Design review of the part built by this model. Coordinates are the model's own, in mm. A direction names the side the tool comes from. Give positions to 0.01 mm unless a question says otherwise; leave off trailing zeros. Loops run counter-clockwise (first coordinate to the right, second up) from the corner with the lowest first, then second, coordinate; pieces in that order, holes last. Notation, with made-up numbers: (4, 37) - (21, 37) arc R20 ccw to (21, 62) - close; hole circle Ø3 at (-3.75, 7.5). An arc over 180 degrees is marked (long way). One line per item, written item: value. Start each with the question number.
```python
from build123d import *

# Parameters (mm, degrees)
SKETCH1_R           = 1.4
BOSS_EXTRUDE1_DEPTH = 3


with BuildPart() as part:
    # Sketch1 → Boss-Extrude1 (new body)
    with BuildSketch(Plane(origin=(0, 0, 0), x_dir=(1, 0, 0), z_dir=(0, 1, 0))):
        with BuildLine():
            Line((-6.037453791, -13.924683413), (-12.047861431, -7.914275773))
            ThreePointArc((-12.047861431, -7.914275773), (-12.926541087, -5.792955429), (-12.047861431, -3.671635086))
            Line((-12.047861431, -3.671635086), (8.458235223, 16.834461569))
            ThreePointArc((8.458235223, 16.834461569), (10.579555567, 17.713141225), (12.700875911, 16.834461569))
            Line((12.700875911, 16.834461569), (18.711283551, 10.824053929))
            ThreePointArc((18.711283551, 10.824053929), (19.418390332, 10.53116071), (20.125497113, 10.824053929))
            Line((20.125497113, 10.824053929), (25.075244581, 15.773801397))
            Line((25.075244581, 15.773801397), (17.606467502, 23.242578477))
            ThreePointArc((17.606467502, 23.242578477), (15.984350757, 24.326442233), (14.070933596, 24.707044571))
            Line((14.070933596, 24.707044571), (7.088177538, 24.707044571))
            ThreePointArc((7.088177538, 24.707044571), (5.174760376, 24.326442233), (3.552643632, 23.242578477))
            Line((3.552643632, 23.242578477), (-18.455978339, 1.233956505))
            ThreePointArc((-18.455978339, 1.233956505), (-19.539842096, -0.388160239), (-19.920444433, -2.301577401))
            Line((-19.920444433, -2.301577401), (-19.920444433, -9.284333458))
            ThreePointArc((-19.920444433, -9.284333458), (-19.539842096, -11.19775062), (-18.455978339, -12.819867364))
            Line((-18.455978339, -12.819867364), (-10.987201259, -20.288644444))
            Line((-10.987201259, -20.288644444), (-6.037453791, -15.338896975))
            ThreePointArc((-6.037453791, -15.338896975), (-5.744560572, -14.631790194), (-6.037453791, -13.924683413))
        make_face()
        with Locations((18.711283551, 16.480908178)):
            Circle(SKETCH1_R, mode=Mode.SUBTRACT)
        with Locations((2.447827583, 16.480908178)):
            Circle(SKETCH1_R, mode=Mode.SUBTRACT)
        with Locations((-11.69430804, 2.338772554)):
            Circle(SKETCH1_R, mode=Mode.SUBTRACT)
        with Locations((-11.69430804, -13.924683413)):
            Circle(SKETCH1_R, mode=Mode.SUBTRACT)
    extrude(amount=BOSS_EXTRUDE1_DEPTH)


solid = part.part
```
(1) Take a section at D-D on z = 8.5. State the section outline as (x, y) points.
(2) Take a section at C-C on y = 0.5. State the section outline as (x, z) points.
(3) Draft analysis for pull direction Z (two halves, no side actions). For faces 1 (the flat face through (-14.774, 1.479, 16.502)), 2 (the cylindrical face through (-12.926, 1.479, 5.826)), 3 (the cylindrical face through (-13.093, 1.479, -2.4)), 4 (the flat face through (-3, 3, -7)), state which applies: pulls with the +Z half, pulls with the -Z half, needs draft (parallel to the pull), parting line crosses it, or undercut.
(4) Take a section at A-A on x = 19.5. State the section outline as (y, z) points.
(5) Take a section at B-B on z = -3. State the section outline as (x, y) points, and give its area (3 significant figures).
(6) For pin 1 Ø4.5 at (x, z) = (-11.69, 13.92) entering from +Y; pin 2 Ø1.7 at (x, z) = (2.45, -16.48) entering from +Y, all flat-tipped, find the tip position at first contact; note any pin that passes through.
(7) To check wall thickness, follow L1, parallel to X at y = 0.2, z = -15.5; L2, parallel to X at y = 1.1, z = -1.5; L3, parallel to Z at x = 18, y = 0.6. State the ranges of each line that lie inside material, in increasing order. Write a range as from..to.
(8) Machinability: for faces 5 (the flat face through (-1.938, 1.479, -6.438)), 6 (the flat face through (15.664, 1.479, -13.871)), 7 (the flat face through (-9, 1.48, 10.96)), which of the approach directions +Z, -Z, +X, -X, +Y, -Y give a long, thin tool a straight path to every point of the face, cutting with its end or side? Answer none if there is none.
Here are the results:
1. outline: (-19.92, 0) - (-11.46, 0) - (-11.46, 3) - (-19.92, 3) - close
2. outline: (-19.92, 2.3) arc R5 ccw to (-18.46, -1.23) - (3.55, -23.24) arc R5 ccw to (7.09, -24.71) - (14.07, -24.71) arc R5 ccw to (17.61, -23.24) - (25.08, -15.77) - (20.13, -10.82) arc R1 ccw to (18.71, -10.82) - (12.7, -16.83) arc R3 cw to (8.46, -16.83) - (-12.05, 3.67) arc R3 cw to (-12.05, 7.91) - (-6.04, 13.92) arc R1 ccw to (-6.04, 15.34) - (-10.99, 20.29) - (-18.46, 12.82) arc R5 ccw to (-19.92, 9.28) - close; hole circle Ø2.8 at (-11.69, -2.34); hole circle Ø2.8 at (-11.69, 13.92); hole circle Ø2.8 at (2.45, -16.48); hole circle Ø2.8 at (18.71, -16.48)
3. face 1: pulls with the +Z half
3. face 2: undercut
3. face 3: undercut
3. face 4: needs draft
4. outline: (0, -21.35) - (3, -21.35) - (3, -17.64) - (0, -17.64) - close; (0, -15.32) - (3, -15.32) - (3, -10.53) - (0, -10.53) - close
5. outline: (-16.69, 0) - (-12.93, 0) - (-12.93, 3) - (-16.69, 3) - close; (-10.46, 0) - (-5.38, 0) - (-5.38, 3) - (-10.46, 3) - close
5. area: 26.5 mm²
6. pin 1: y = 3
6. pin 2: through
7. L1: -4.19..1.45, 3.45..7.12, 14.04..17.71, 19.71..24.8
7. L2: -18.19..-12.82, -10.57..-6.88
7. L3: -22.85..-17.69, -15.28..-11.54
8. face 5: +Y, -Y
8. face 6: +Z, +Y, -Y
8. face 7: +X, +Y, -Y
